```python
from build123d import *

# Parameters (mm, degrees)
F1_DEPTH = 63.5
F2_DEPTH = 25.4
F3_DEPTH = 7.9375
F4_DEPTH = 25.4


with BuildPart() as f1:
    # F0 (on Front) → F1 (new body, symmetric)
    with BuildSketch(Plane.XZ):
        Polygon((41.275, -9.525), (41.275, 9.525), (22.225, 9.525), (-41.275, 9.525), (-41.275, -9.525), align=None)
    extrude(amount=F1_DEPTH, both=True)

    # F0 (on Front) → F2 (join, symmetric)
    with BuildSketch(Plane.XZ):
        with BuildLine():
            Line((22.225, 9.525), (41.275, 9.525))
            Line((41.275, 9.525), (41.275, 25.4))
            ThreePointArc((41.275, 25.4), (45.92468, 36.62532), (57.15, 41.275))
            Line((57.15, 41.275), (63.898031, 41.275))
            Line((63.898031, 41.275), (63.898031, 60.325))
            add(Edge.make_bspline(
                [(47.724872, 59.029193), (52.819319, 59.523847), (58.204508, 59.955469), (63.898031, 60.325)],
                knots=[108.105541, 108.105541, 108.105541, 108.105541, 116.799, 116.799, 116.799, 116.799], degree=3))
            ThreePointArc((47.724872, 59.029193), (29.320805, 46.501932), (22.225, 25.4))
            Line((22.225, 25.4), (22.225, 9.525))
        make_face()
    extrude(amount=F2_DEPTH, both=True)

    # F0 (on Front) → F3 (join, symmetric)
    with BuildSketch(Plane.XZ):
        with BuildLine():
            Line((-41.275, 9.525), (22.225, 9.525))
            Line((22.225, 9.525), (22.225, 25.4))
            ThreePointArc((22.225, 25.4), (29.320805, 46.501932), (47.724872, 59.029193))
            add(Edge.make_bspline(
                [(-41.275, 9.525), (-34.017475, 36.97978), (-15.625963, 52.878028), (47.724872, 59.029193)],
                knots=[0, 0, 0, 0, 108.105541, 108.105541, 108.105541, 108.105541], degree=3))
        make_face()
    extrude(amount=F3_DEPTH, both=True)

    # F2_face (on face) → F4 (join)
    with BuildSketch(Plane(origin=(63.898031, 0, 50.8), x_dir=(0, 1, 0), z_dir=(1, 0, 0))):
        Polygon((25.4, -9.525), (25.4, 9.525), (0, 9.525), (-25.4, 9.525), (-25.4, -9.525), align=None)
    extrude(amount=F4_DEPTH)


solid = f1.part
```
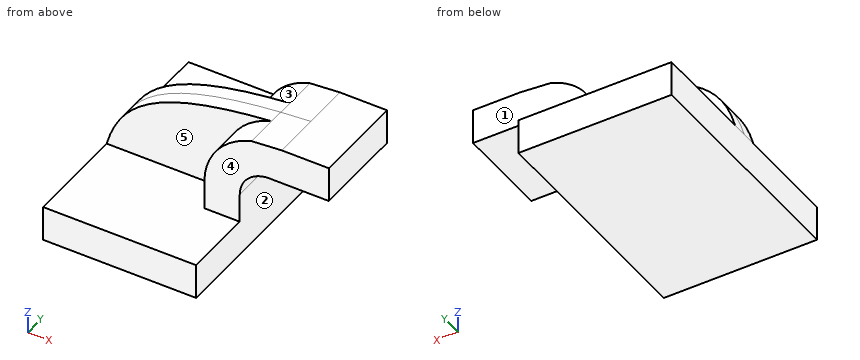
Source: CAD feature listing. Evaluate the final solid. Frame: model axes, mm. Face numbers are marked on the shaded views. A direction names the side the tool comes from. Coordinates: 2 decimals unless noted, no trailing zeros. Loops run counter-clockwise (first coordinate to the right, second up) from the corner with the lowest first, then second, coordinate; pieces in that order, holes last. Notation, with made-up numbers: (38.25, 17) -> (90.25, 17) arc R15 ccw to (90.25, 28) -> close; hole circle Ø4 at (72, -27.5). An arc over 180 degrees is marked (long way). One line per item, written item: value. Start each with the question number.
Q1. Set-up query: the marked faces 1, 2, 3, 4 and 5. Return all of +Z, -Z, +X, -X, +Y, -Y with unobstructed straight access to the full face (end or side cutting, diameter ignored); none if empty.
Q2. Section query A-A, the plane x = 80.5. Return the cut outline in (y, z) (3 decimals), and give its area (3 significant figures).
Q3. Line query: line 1 along Y through (x, z) = (33, 24); line 2 along X through (y, z) = (13, 3.5) (3 decimals); line 3 along Y through (x, z) = (-30, 28.5). Output: solid intervals per line, ascending.
Q4. Section query B-B, the plane y = -49. Return the cut outline in (x, z) (3 decimals).
Q5. Contact query for flat-ended pins moving along their axis: P1, Ø15, axis at x = 40, z = 33, coming from the -Y side; P2, Ø12, axis at x = 76, y = -3, coming from the -Z side (3 decimals); P3, Ø4, axis at x = 47.5, y = 11, coming from the +Z side; P4, Ø12, axis at x = 59.5, y = 4, coming from the +Z side (3 decimals). Output: stop coordinate, or through.
Results:
1. face 1: +Z, +X, -X, +Y
1. face 2: -Z, +X, +Y, -Y
1. face 3: +Z, -X, +Y
1. face 4: +Z, +X, -X, -Y
1. face 5: +Z, -X, -Y
2. outline: (-25.4, 41.275) -> (25.4, 41.275) -> (25.4, 60.325) -> (-25.4, 60.325) -> close
2. area: 968 mm^2
3. line 1: -25.4 to 25.4
3. line 2: -41.275 to 41.275
3. line 3: -7.94 to 7.94
4. outline: (-41.275, -9.525) -> (41.275, -9.525) -> (41.275, 9.525) -> (-41.275, 9.525) -> close
5. P1: y = -25.4
5. P2: z = 41.275
5. P3: z = 59.2
5. P4: z = 60.325
